Read the model definition and answer for the solid it produces. Units are mm, in the model's axes. Face numbers are marked on the shaded views. A direction names the side the tool comes from. Coordinates: 2 decimals unless noted, no trailing zeros. Write each loop counter-clockwise with the first axis right and the second up, starting at its lowest first coordinate (ties: lowest second). Pieces come first, ordered by that corner, then holes.
1) The part is cut by section A-A (y = 27.5). Determine the outline of the cut face in (x, z) (3 decimals).
2) Determine the mould class of the marked faces 4, 5 and 6 for opening direction X: +X half, -X half, draft (parallel to the pull), parting line (faces both ways), or undercut.
3) Which of the six approach directions +Z, -Z, +X, -X, +Y, -Y give full straight-line access (tool end or side, diameter ignored) to the marked faces 1, 2 and 3?
4) Find the intervals of material crossed by line 1 (Y direction, x = 205.5, z = -35.5) (3 decimals); line 2 (Y direction, x = 107, z = -38); line 3 (X direction, y = -15.5, z = 12), in increasing order.
5) The part is cut by section D-D (z = 0). Determine the outline of the cut face in (x, y) (3 decimals), then the cut area to 3 significant figures.
6) Each of these flat-tipped pins is pushed along its axis until it touches: pin 1 Ø1.5 at (y, z) = (28.5, -12.5) entering from +X (3 decimals); pin 2 Ø3 at (x, y) = (96.5, -9) entering from -Z; pin 3 Ø8 at (x, y) = (161, 10.5) entering from -Z. Where does it stop, or does it pass through?
7) The part is cut by section B-B (y = 60). Determine the outline of the cut face in (x, z).
8) The part is cut by section C-C (x = 143). Determine the outline of the cut face in (y, z) (3 decimals), then the cut area to 3 significant figures.
from build123d import *

# Parameters (mm, degrees)
BOSS_EXTRUDE2_DEPTH      = 63.5
BOSS_EXTRUDE2_DEPTH_BACK = 63.5
SKETCH3_R                = 46.99
BOSS_EXTRUDE3_DEPTH      = 6.35
CUT_EXTRUDE1_DEPTH       = 31.115
CUT_EXTRUDE1_DEPTH_BACK  = 31.115
BOSS_EXTRUDE4_DEPTH      = 31.115
BOSS_EXTRUDE4_DEPTH_BACK = 31.115
SKETCH5_R                = 22.225


with BuildPart() as part:
    # Sketch2 → Boss-Extrude2 (new, two sides: drawn at the far end of the back side and taken through both)
    with BuildSketch(Plane(origin=(0, 0, 0), x_dir=(0, 0, -1), z_dir=(0, 1, 0)).offset(-BOSS_EXTRUDE2_DEPTH_BACK)):
        with BuildLine():
            Line((-107.95, -38.1), (-107.95, -155.921006071))
            ThreePointArc((-107.95, -155.921006071), (-104.47415367, -170.365199862), (-94.807654535, -181.646823701))
            Line((-94.807654535, -181.646823701), (-22.329185441, -234.070981156))
            ThreePointArc((-22.329185441, -234.070981156), (17.333032549, -237.128984404), (38.1, -203.2))
            Line((38.1, -203.2), (38.1, -27.503637941))
            ThreePointArc((38.1, -27.503637941), (32.92252616, 33.528605269), (-28.194, 37.592))
            Line((-28.194, 37.592), (-95.25, -12.7))
            ThreePointArc((-95.25, -12.7), (-104.598063314, -23.900968343), (-107.95, -38.1))
        make_face()
    extrude(amount=BOSS_EXTRUDE2_DEPTH + BOSS_EXTRUDE2_DEPTH_BACK)

    # Sketch3 → Boss-Extrude3 (add)
    with BuildSketch(Plane(origin=(0, 63.5, 0), x_dir=(1, 0, 0), z_dir=(0, 1, 0))):
        with Locations(Location((0, 0, 0), (0, 0, 270))):
            Circle(SKETCH3_R)
    extrude(amount=BOSS_EXTRUDE3_DEPTH)

    # Sketch4 → Cut-Extrude1 (cut, two sides: drawn at the far end of the back side and taken through both)
    with BuildSketch(Plane(origin=(0, 0, 0), x_dir=(1, 0, 0), z_dir=(0, 1, 0)).offset(-CUT_EXTRUDE1_DEPTH_BACK)):
        with BuildLine():
            Line((125.379811821, 38.1), (277.779811821, 38.1))
            Line((277.779811821, 38.1), (188.463070055, -85.383924623))
            ThreePointArc((188.463070055, -85.383924623), (142.063874206, -31.232130195), (125.379811821, 38.1))
        make_face()
    extrude(amount=CUT_EXTRUDE1_DEPTH + CUT_EXTRUDE1_DEPTH_BACK, mode=Mode.SUBTRACT)

    # Sketch5 → Boss-Extrude4 (add, two sides: drawn at the far end of the back side and taken through both)
    with BuildSketch(Plane(origin=(0, 0, 0), x_dir=(1, 0, 0), z_dir=(0, 1, 0)).offset(-BOSS_EXTRUDE4_DEPTH_BACK)):
        with Locations(Location((203.2, 0, 0), (0, 0, 270))):
            Circle(SKETCH5_R)
    extrude(amount=BOSS_EXTRUDE4_DEPTH + BOSS_EXTRUDE4_DEPTH_BACK)


solid = part.part
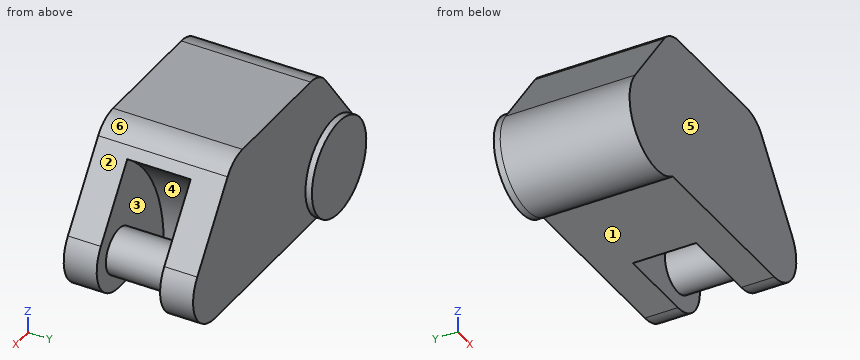
Reported:
1. outline: (-37.592, 28.194) arc R46.99 ccw to (27.504, -38.1) - (125.38, -38.1) arc R152.4 cw to (188.463, 85.384) - (181.647, 94.808) arc R31.75 ccw to (155.921, 107.95) - (38.1, 107.95) arc R31.75 ccw to (12.7, 95.25) - close; circle Ø44.45 at (203.2, 0)
2. face 4: undercut
2. face 5: draft
2. face 6: +X half
3. face 1: -Z, +X, +Y, -Y
3. face 2: +Z, +X, +Y, -Y
3. face 3: none
4. line 1: y = -63.5 to -31.115, 31.115 to 63.5
4. line 2: y = -63.5 to 63.5
4. line 3: x = -45.43 to 133.85, 184.49 to 221.91
5. outline: (-46.99, -63.5) - (241.3, -63.5) - (241.3, -31.115) - (225.425, -31.115) - (225.425, 31.115) - (241.3, 31.115) - (241.3, 63.5) - (46.99, 63.5) - (46.99, 69.85) - (-46.99, 69.85) - close; hole (130.219, -31.115) - (180.975, -31.115) - (180.975, 31.115) - (130.219, 31.115) - close
5. area: 33,100 mm2
6. pin 1: stops at x = 222.065
6. pin 2: stops at z = -38.1
6. pin 3: stops at z = 54.84
7. outline: (-37.59, 28.19) arc R46.99 ccw to (27.5, -38.1) - (203.2, -38.1) arc R38.1 ccw to (234.07, 22.33) - (181.65, 94.81) arc R31.75 ccw to (155.92, 107.95) - (38.1, 107.95) arc R31.75 ccw to (12.7, 95.25) - close
8. outline: (-63.5, -38.1) - (-31.115, -38.1) - (-31.115, 33.035) - (31.115, 33.035) - (31.115, -38.1) - (63.5, -38.1) - (63.5, 107.95) - (-63.5, 107.95) - close
8. area: 14,100 mm2
